Source: CAD feature listing. Evaluate the final solid. Frame: model axes, mm. Coordinates: 2 decimals unless noted, no trailing zeros. Order: outer loops, then holes, each group sorted by start corner. A loop starts at its lowest first (then second) coordinate and runs counter-clockwise, first axis right, second up. Notation, with made-up numbers: (26, -8.75) -> (85, -8.75) arc R29 ccw to (85, 23.25) -> close; hole circle Ø10 at (78.5, -10.75). An arc over 180 degrees is marked (long way). Put each result on its own line as item: value.
from build123d import *

# Parameters (mm, degrees)
SKETCH2_R           = 15
BOSS_EXTRUDE1_DEPTH = 5


with BuildPart() as part:
    # Sketch2 → Boss-Extrude1 (new, symmetric)
    with BuildSketch(Plane.XY):
        with BuildLine():
            ThreePointArc((-22.73046694, 29.636563105), (-18.64010484, 27.256433461), (-19.682902282, 22.640303835))
            ThreePointArc((-19.682902282, 22.640303835), (-21.213203436, 21.213203436), (-22.640303835, 19.682902282))
            ThreePointArc((-22.640303835, 19.682902282), (-27.256433461, 18.64010484), (-29.636563105, 22.73046694))
            ThreePointArc((-29.636563105, 22.73046694), (-37.853751933, 35.41031558), (-51.961524227, 30))
            ThreePointArc((-51.961524227, 30), (-60, 0), (-51.961524227, -30))
            ThreePointArc((-51.961524227, -30), (-37.853751933, -35.41031558), (-29.636563105, -22.73046694))
            ThreePointArc((-29.636563105, -22.73046694), (-27.256433461, -18.64010484), (-22.640303835, -19.682902282))
            ThreePointArc((-22.640303835, -19.682902282), (-21.213203436, -21.213203436), (-19.682902282, -22.640303835))
            ThreePointArc((-19.682902282, -22.640303835), (-18.64010484, -27.256433461), (-22.73046694, -29.636563105))
            ThreePointArc((-22.73046694, -29.636563105), (-35.41031558, -37.853751933), (-30, -51.961524227))
            ThreePointArc((-30, -51.961524227), (0, -60), (30, -51.961524227))
            ThreePointArc((30, -51.961524227), (35.41031558, -37.853751933), (22.73046694, -29.636563105))
            ThreePointArc((22.73046694, -29.636563105), (18.64010484, -27.256433461), (19.682902282, -22.640303835))
            ThreePointArc((19.682902282, -22.640303835), (21.213203436, -21.213203436), (22.640303835, -19.682902282))
            ThreePointArc((22.640303835, -19.682902282), (27.256433461, -18.64010484), (29.636563105, -22.73046694))
            ThreePointArc((29.636563105, -22.73046694), (37.853751933, -35.41031558), (51.961524227, -30))
            ThreePointArc((51.961524227, -30), (60, 0), (51.961524227, 30))
            ThreePointArc((51.961524227, 30), (37.853751933, 35.41031558), (29.636563105, 22.73046694))
            ThreePointArc((29.636563105, 22.73046694), (27.256433461, 18.64010484), (22.640303835, 19.682902282))
            ThreePointArc((22.640303835, 19.682902282), (21.213203436, 21.213203436), (19.682902282, 22.640303835))
            ThreePointArc((19.682902282, 22.640303835), (18.64010484, 27.256433461), (22.73046694, 29.636563105))
            ThreePointArc((22.73046694, 29.636563105), (35.41031558, 37.853751933), (30, 51.961524227))
            ThreePointArc((30, 51.961524227), (0, 60), (-30, 51.961524227))
            ThreePointArc((-30, 51.961524227), (-35.41031558, 37.853751933), (-22.73046694, 29.636563105))
        make_face()
        Circle(SKETCH2_R, mode=Mode.SUBTRACT)
        with BuildLine():
            ThreePointArc((-21, 36.373066959), (-29.196152423, 38.569219382), (-27, 46.765371804))
            ThreePointArc((-27, 46.765371804), (0, 54), (27, 46.765371804))
            ThreePointArc((27, 46.765371804), (29.196152423, 38.569219382), (21, 36.373066959))
            ThreePointArc((21, 36.373066959), (0, 42), (-21, 36.373066959))
        make_face(mode=Mode.SUBTRACT)
        with BuildLine():
            ThreePointArc((-46.765371804, 27), (-38.569219382, 29.196152423), (-36.373066959, 21))
            ThreePointArc((-36.373066959, 21), (-42, 0), (-36.373066959, -21))
            ThreePointArc((-36.373066959, -21), (-38.569219382, -29.196152423), (-46.765371804, -27))
            ThreePointArc((-46.765371804, -27), (-54, 0), (-46.765371804, 27))
        make_face(mode=Mode.SUBTRACT)
        with BuildLine():
            ThreePointArc((46.765371804, -27), (38.569219382, -29.196152423), (36.373066959, -21))
            ThreePointArc((36.373066959, -21), (42, 0), (36.373066959, 21))
            ThreePointArc((36.373066959, 21), (38.569219382, 29.196152423), (46.765371804, 27))
            ThreePointArc((46.765371804, 27), (54, 0), (46.765371804, -27))
        make_face(mode=Mode.SUBTRACT)
        with BuildLine():
            ThreePointArc((-27, -46.765371804), (-29.196152423, -38.569219382), (-21, -36.373066959))
            ThreePointArc((-21, -36.373066959), (0, -42), (21, -36.373066959))
            ThreePointArc((21, -36.373066959), (29.196152423, -38.569219382), (27, -46.765371804))
            ThreePointArc((27, -46.765371804), (0, -54), (-27, -46.765371804))
        make_face(mode=Mode.SUBTRACT)
    extrude(amount=BOSS_EXTRUDE1_DEPTH, both=True)


solid = part.part
1. Pull-direction query (X, two-part tool) for faces 1 (the cylindrical face through (-60, 0, 0)), 2 (the cylindrical face through (0, -60, 0)), 3 (the cylindrical face through (-54, 0, 0)), 4 (the cylindrical face through (37.64, -35.34, 0.07)); classes: pulls with the +X half, pulls with the -X half, needs draft (parallel to the pull), parting line crosses it, or undercut.
Numbers:
face 1: pulls with the -X half
face 2: parting line crosses it
face 3: undercut
face 4: undercut
2. First-contact query: pin 1 (5 mm diameter, centred on y = -25, z = -3, fed in from -X); pin 2 (1 mm diameter, centred on x = -44, z = 0.5, fed in from +Y); pin 3 (1.5 mm diameter, centred on x = 28, z = -4, fed in from -Y) (3 decimals). Flat tips, straight axial feed; report the tip coordinate or a pass-through.
Numbers:
pin 1: stops at x = -55.62
pin 2: stops at y = 35.84
pin 3: stops at y = -53.455
3. Cut plane A-A on y = 0. Output: boundary loops of the cut face in (x, z).
Numbers:
outline: (-60, -5) -> (-54, -5) -> (-54, 5) -> (-60, 5) -> close; (-42, -5) -> (-15, -5) -> (-15, 5) -> (-42, 5) -> close; (15, -5) -> (42, -5) -> (42, 5) -> (15, 5) -> close; (54, -5) -> (60, -5) -> (60, 5) -> (54, 5) -> close
4. Ray query, line 1 along Y through (x, z) = (0, -2); line 2 along X through (y, z) = (36.5, -1.5); line 3 along Y through (x, z) = (-24, 2). Return the intervals inside material, ascending.
Numbers:
line 1: y = -60 to -54, -42 to -15, 15 to 42, 54 to 60
line 2: x = -34.88 to -27.21, -20.78 to 20.78, 27.21 to 34.88
line 3: y = -54.99 to -48.37, -35.57 to -29.57, -18.67 to 18.67, 29.57 to 35.57, 48.37 to 54.99
5. Cut plane D-D on y = -24.5. Output: boundary loops of the cut face in (x, z).
Numbers:
outline: (-54.77, -5) -> (-48.12, -5) -> (-48.12, 5) -> (-54.77, 5) -> close; (-35.59, -5) -> (-29.58, -5) -> (-29.58, 5) -> (-35.59, 5) -> close; (-18.48, -5) -> (18.48, -5) -> (18.48, 5) -> (-18.48, 5) -> close; (29.58, -5) -> (35.59, -5) -> (35.59, 5) -> (29.58, 5) -> close; (48.12, -5) -> (54.77, -5) -> (54.77, 5) -> (48.12, 5) -> close
6. Cut plane C-C on x = 44. Output: boundary loops of the cut face in (y, z), plus the area to 3 significant figures.
Numbers:
outline: (-35.75, -5) -> (-29.49, -5) -> (-29.49, 5) -> (-35.75, 5) -> close; (29.49, -5) -> (35.75, -5) -> (35.75, 5) -> (29.49, 5) -> close
area: 125 mm2
